from build123d import *

# Parameters (mm, degrees)
SKETCH1_W                    = 50.8
SKETCH1_H                    = 6.35
BOSS_EXTRUDE1_DEPTH          = 5.08
F_10_0_1935_DIAMETER_HOLE1_D = 4.9149
F_1_8_0_1250_DOWEL_HOLE1_D   = 3.175
CUT_EXTRUDE1_DEPTH           = 56.613276798
FILLET1_R                    = 3.81


with BuildPart() as part:
    # Sketch1 → Boss-Extrude1 (new body)
    with BuildSketch(Plane(origin=(0, 0, 0), x_dir=(1, 0, 0), z_dir=(0, 1, 0))):
        with BuildLine():
            Line((25.4, -6.35), (-25.4, -6.35))
            Line((-25.4, -6.35), (-25.4, -9.980909488))
            Line((-25.4, -9.980909488), (-4.124445986, -46.83125))
            ThreePointArc((-4.124445986, -46.83125), (0, -49.2125), (4.124445986, -46.83125))
            Line((4.124445986, -46.83125), (25.4, -9.980909488))
            Line((25.4, -9.980909488), (25.4, -6.35))
        make_face()
        with Locations((0, -3.175)):
            Rectangle(SKETCH1_W, SKETCH1_H)
    extrude(amount=BOSS_EXTRUDE1_DEPTH)

    # #10 (0.1935) Diameter Hole1 (through all)
    with Locations(Plane(origin=(0, 5.08, 0), x_dir=(1, 0, 0), z_dir=(0, 1, 0))):
        with Locations((-12.7, -6.35), (12.7, -6.35)):
            Hole(F_10_0_1935_DIAMETER_HOLE1_D / 2)

    # 1/8 (0.1250) Dowel Hole1 (through all)
    with Locations(Plane(origin=(0, 5.08, 0), x_dir=(1, 0, 0), z_dir=(0, 1, 0))):
        with Locations((0, -44.45)):
            Hole(F_1_8_0_1250_DOWEL_HOLE1_D / 2)

    # Sketch4 → Cut-Extrude1 (cut, through all)
    with BuildSketch(Plane(origin=(0, 5.08, 0), x_dir=(1, 0, 0), z_dir=(0, 1, 0))):
        with BuildLine():
            Line((-6.027562939, -3.175), (-9.070487533, -8.4455))
            ThreePointArc((-9.070487533, -8.4455), (-9.73651548, -9.31348452), (-10.6045, -9.979512467))
            Line((-10.6045, -9.979512467), (-18.952099271, -14.799001153))
            Line((-18.952099271, -14.799001153), (-11.799907664, -27.186960401))
            Line((-11.799907664, -27.186960401), (-7.506626388, -34.623141702))
            add(Edge.make_bspline(
                [(7.506626388, -34.623141702), (5.246523419, -38.15236124), (0, -44.39763876), (-5.246523419, -38.15236124), (-7.506626388, -34.623141702)],
                knots=[0.213351666, 0.213351666, 0.213351666, 0.213351666, 0.5, 0.786648334, 0.786648334, 0.786648334, 0.786648334], degree=3))
            Line((7.506626388, -34.623141702), (11.799907664, -27.186960401))
            Line((11.799907664, -27.186960401), (18.952099271, -14.799001153))
            Line((18.952099271, -14.799001153), (10.6045, -9.979512467))
            ThreePointArc((10.6045, -9.979512467), (9.73651548, -9.31348452), (9.070487533, -8.4455))
            Line((9.070487533, -8.4455), (6.027562939, -3.175))
            Line((6.027562939, -3.175), (-6.027562939, -3.175))
        make_face()
    extrude(amount=-CUT_EXTRUDE1_DEPTH, mode=Mode.SUBTRACT)

    # Fillet1
    fillet1_edges = [part.edges().sort_by_distance(p)[0] for p in [
        (-25.4, 2.54, 9.980909488),
        (-25.4, 2.54, 0),
        (25.4, 2.54, 0),
        (25.4, 2.54, 9.980909488),
        (-18.952099271, 2.54, 14.799001153),
        (-6.027562939, 2.54, 3.175),
        (6.027562939, 2.54, 3.175),
        (18.952099271, 2.54, 14.799001153),
    ]]
    fillet(fillet1_edges, radius=FILLET1_R)


solid = part.part
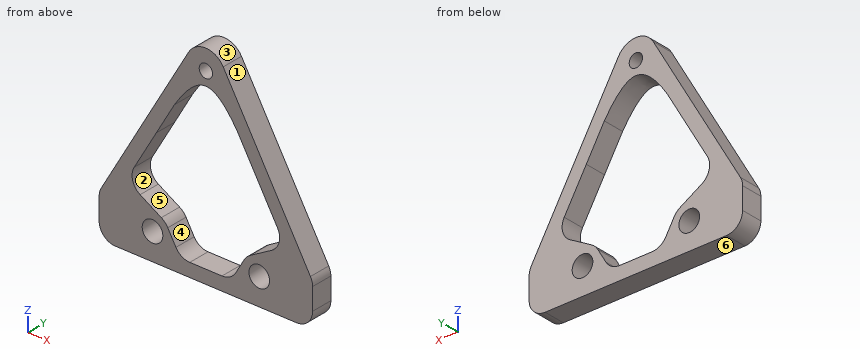
CAD build for the part. Positions are in the model's coordinates, mm. Face numbers are marked on the shaded views. A direction names the side the tool comes from. Give positions to 0.01 mm unless a question says otherwise; leave off trailing zeros. Write each loop counter-clockwise with the first axis right and the second up, starting at its lowest first coordinate (ties: lowest second). Pieces come first, ordered by that corner, then holes. Notation, with made-up numbers: M 37,-36.75 L 82,-36.75 A26 ccw 82,-4.75 Z; hole C 70.25,7 d1. An arc over 180 degrees is marked long. Put each result on its own line as item: value. Start each with the question number.
(1) Flat gauge pins, fed straight in: pin 1 Ø1.5 at (y, z) = (3.5, 21) entering from -X; pin 2 Ø1.5 at (x, y) = (-1.5, 3) entering from +Z; pin 3 Ø4.5 at (x, z) = (12.7, 6.35) entering from +Y. Where does each tip first touch, or does it go through?
(2) Band-saw the part on B-B, the plane z = 26. Write the cut outline in (x, y), and give its area (3 significant figures).
(3) Probe L1, parallel to Z at x = 12, y = 1.85; L2, parallel to X at y = 0.4, z = 6.5; L3, parallel to Z at x = -13.5, y = 3.8. List the from-to ranges inside material, lowest first.
(4) Band-saw the part on D-D, the plane y = 4. Give the number of separate pieces and of enclosed holes in the cut face, and give its area (3 significant figures).
(5) Mould opens along Z. For the marked faces 3, 4, 5 and 6 say: +Z half, -Z half, draft (parallel to the pull), parting line (faces both ways), or undercut.
(6) Band-saw the part on C-C, the plane z = 6.35. Write the cut outline in (x, y), and give its area (3 significant figures).
(7) Which spindle directions (+Z, -Z, +X, -X, +Y, -Y) get a long thin tool onto all of the face, cutting with end or side? Do the marked faces 1 and 2. Say none if no direction does.
(8) Band-saw the part on A-A, the plane x = -14. Write the cut outline in (y, z).
Response values:
1. pin 1: stops at x = -19.47
1. pin 2: stops at z = 49.15
1. pin 3: passes through
2. outline: M -16.15,0 L -12.49,0 L -12.49,5.08 L -16.15,5.08 Z; M 12.49,0 L 16.15,0 L 16.15,5.08 L 12.49,5.08 Z
2. area: 37.2 mm2
3. L1: z = 0 to 3.99, 8.71 to 10.79, 26.84 to 33.19
3. L2: x = -25.4 to -15.15, -10.25 to -7.95, 7.95 to 10.25, 15.15 to 25.4
3. L3: z = 0 to 4.03, 8.67 to 11.65, 24.24 to 30.59
4. separate pieces: 1
4. enclosed holes: 4
4. area: 724 mm2
5. face 3: +Z half
5. face 4: undercut
5. face 5: undercut
5. face 6: -Z half
6. outline: M -25.4,0 L -15.16,0 L -15.16,5.08 L -25.4,5.08 Z; M -10.24,0 L -7.86,0 L -7.86,5.08 L -10.24,5.08 Z; M 7.86,0 L 10.24,0 L 10.24,5.08 L 7.86,5.08 Z; M 15.16,0 L 25.4,0 L 25.4,5.08 L 15.16,5.08 Z
6. area: 128 mm2
7. face 1: +Z, +X, +Y, -Y
7. face 2: +Y, -Y
8. outline: M 0,0 L 5.08,0 L 5.08,4.26 L 0,4.26 Z; M 0,8.44 L 5.08,8.44 L 5.08,11.94 L 0,11.94 Z; M 0,23.38 L 5.08,23.38 L 5.08,29.73 L 0,29.73 Z
